The model under review builds one solid part; all positions refer to its coordinate system, in mm. Coordinates: 2 decimals unless noted, no trailing zeros. Order: outer loops, then holes, each group sorted by start corner. A loop starts at its lowest first (then second) coordinate and runs counter-clockwise, first axis right, second up. Notation, with made-up numbers: M 67,32 L 88,32 A28 ccw 88,69 Z; hole C -35,-15.75 d6. An arc over 180 degrees is marked long. Answer as CSV lines item,"result". Start each with the question number.
Q1. For P1, Ø1.5, axis at y = 1.5, z = 1.5, coming from the -X side; P2, Ø1.5, axis at y = -6, z = 2, coming from the -X side, all flat-tipped, find the tip position at first contact; note any pin that passes through.
Q2. Consider section B-B on z = 2. Write out the cut boundary in (x, y).
Q3. Wall thickness on L1, parallel to Y at x = 0, z = 0.7; L2, parallel to Y at x = -150, z = 1.7; L3, parallel to X at y = -1.5, z = 4.35: over which ranges is each line inside the solid? List them lowest first. Write a range as [from, to].
Q4. Consider section A-A on y = 0. Write out the cut boundary in (x, z).
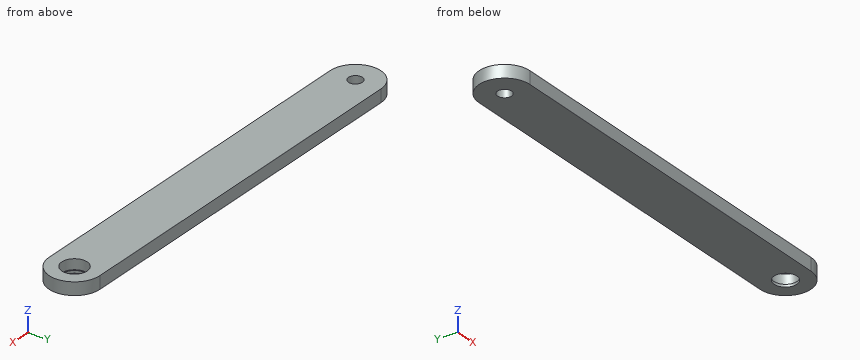
Autodesk Inventor part; units mm, degrees
ref_plane "YZ Plane" through (0, 0, 0) normal (1, 0, 0) x (0, 1, 0)
ref_plane "XZ Plane" through (0, 0, 0) normal (0, 1, 0) x (-1, 0, 0)
ref_plane "XY Plane" through (0, 0, 0) normal (0, 0, 1) x (1, 0, 0)
sketch "Skizze3" plane through (0, 0, 0) normal (0, 0, 1) x (1, 0, 0)
  line L0 (0, 0) -> (-150, 0) construction
  line L1 (0, 10) -> (-150, 10)
  line L2 (-150, -10) -> (0, -10)
  arc A0 (0, -10) -> (0, 10) centre (0, 0) ccw
  arc A1 (-150, 10) -> (-150, -10) centre (-150, 0) ccw
  circle A2 centre (0, 0) radius 5
  circle A3 centre (-150, 0) radius 2.75
  circle A4 centre (0, 0) radius 4.5
  point P0 (-75, 0)
  dimension "d4" = 150
  dimension "d5" = 20
  dimension "d6" = 10
  dimension "d7" = 5.5
  dimension "d12" = 9
extrude "Extrusion3" add sketch "Skizze3" along normal blind 5 contours A0 L2 A1 L1
extrude "Extrusion4" add sketch "Skizze3" along normal blind 1 contours A2
properties part number "BT001_trajan20_21" material "Kunststoff, undurchsichtig Schwarz"
Evaluation:
1,P1,"stops at x = -159.97"
1,P2,"stops at x = -158.51"
2,outline,"M -150,-10 L 0,-10 A10 ccw 0,10 L -150,10 A10 ccw Z; hole C -150,0 d5.5; hole C 0,0 d10"
3,L1,"y = [-10, -4.5], [4.5, 10]"
3,L2,"y = [-10, -2.75], [2.75, 10]"
3,L3,"x = [-159.89, -152.3], [-147.7, -4.77], [4.77, 9.89]"
4,outline,"M -160,0 L -152.75,0 L -152.75,5 L -160,5 Z; M -147.25,0 L -4.5,0 L -4.5,1 L -5,1 L -5,5 L -147.25,5 Z; M 4.5,0 L 10,0 L 10,5 L 5,5 L 5,1 L 4.5,1 Z"
